from build123d import *

# Parameters (mm, degrees)
F1_DEPTH = 1.5875
F2_W     = 15.875
F2_H     = 3.175
F3_DEPTH = 2.38125
F5_W     = 12.7
F5_H     = 3.175
F6_DEPTH = 0.79375
F7_R     = 1.5875


# Not quite as in the source:
# - a feature of the source that left no trace in its solid (it failed there, or was rolled back) is left out


with BuildPart() as f1:
    # F0 (on Top) → F1 (new body)
    with BuildSketch(Plane.XY):
        Polygon((28.575, -6.35), (28.575, 6.35), (6.35, 6.35), (4.7625, 12.7), (-4.7625, 12.7), (-6.35, 6.35), (-28.575, 6.35), (-28.575, -6.35), align=None)
    extrude(amount=F1_DEPTH)

    # F2 (on face) → F3 (join)
    with BuildSketch(Plane.XY.offset(1.5875)):
        Rectangle(F2_W, F2_H)
    extrude(amount=F3_DEPTH)

    # F5 (on offset) → F6 (cut)
    with BuildSketch(Plane.XY.offset(2.38125)):
        Rectangle(F5_W, F5_H)
    extrude(amount=-F6_DEPTH, mode=Mode.SUBTRACT)

    # F7
    f7_edges = [f1.edges().sort_by_distance(p)[0] for p in [
        (-28.575, -6.35, 0.79375),
        (28.575, -6.35, 0.79375),
        (28.575, 6.35, 0.79375),
        (4.7625, 12.7, 0.79375),
        (-28.575, 6.35, 0.79375),
        (-4.7625, 12.7, 0.79375),
        (-6.35, 6.35, 0.79375),
        (6.35, 6.35, 0.79375),
    ]]
    fillet(f7_edges, radius=F7_R)


solid = f1.part
The listing builds one solid part. Answer for the finished solid, in the listing's coordinates (mm). A direction names the side the tool comes from. Give positions to 0.01 mm unless a question says otherwise; leave off trailing zeros. Write each loop counter-clockwise with the first axis right and the second up, starting at its lowest first coordinate (ties: lowest second). Pieces come first, ordered by that corner, then holes. Notation, with made-up numbers: (55.25, 35) - (64.25, 35) arc R15 ccw to (64.25, 58) - close; hole circle Ø1 at (-29, 59). An arc over 180 degrees is marked (long way). Use a Markdown table: item, result.
1. A tool of negligible diameter and unlimited length cuts with its end or side. For faces 4 (the flat face through (17, 6.35, 1)), 5 (the flat face through (-17, 6.35, 1)), 6 (the flat face through (0, -1.588, 3)), 7 (the flat face through (-7.938, 0, 3)), from which of +Z, -Z, +X, -X, +Y, -Y can it reach the whole face along a straight path? Write none if from no direction.
Values follow:
| item | result |
|---|---|
| face 4 | +Z, -Z, +X, +Y |
| face 5 | +Z, -Z, -X, +Y |
| face 6 | +Z, +X, -X, -Y |
| face 7 | +Z, -X, +Y, -Y |
2. Find the intervals of material crossed by probe 1 along Y at (x, z) = (-22, 1.25); probe 2 along X at (y, z) = (1, 3.85); probe 3 along Z at (x, y) = (-15.5, -1), in increasing order. Write a range as from..to.
Values follow:
| item | result |
|---|---|
| probe 1 | y = -6.35..6.35 |
| probe 2 | x = -7.94..7.94 |
| probe 3 | z = 0..1.59 |
3. For a pull along X with two mould halves and no side action, classify faces 1 (the flat face through (0, 1.588, 3)), 2 (the flat face through (7.938, 0, 3)), 3 (the flat face through (0, 0, 2.381)) as released by +X, released by -X, zero draft, split by the parting line, or undercut.
Values follow:
| item | result |
|---|---|
| face 1 | zero draft |
| face 2 | released by +X |
| face 3 | undercut |
4. Section D-D on y = 4.25 is taken. Write down the section's boundary in (x, z) (1 decimal), plus the area to 3 significant figures.
Values follow:
| item | result |
|---|---|
| outline | (-28.6, 0) - (28.6, 0) - (28.6, 1.6) - (-28.6, 1.6) - close |
| area | 90.7 mm² |
5. Section A-A on x = -2.5 is taken. Write down the section's boundary in (y, z).
Values follow:
| item | result |
|---|---|
| outline | (-6.35, 0) - (12.7, 0) - (12.7, 1.59) - (-6.35, 1.59) - close; (-1.59, 2.38) - (1.59, 2.38) - (1.59, 3.97) - (-1.59, 3.97) - close |
6. Each of these flat-tipped pins is pushed along its axis until it touches: P1, Ø0.5, axis at x = 19.5, z = 0.5, coming from the +Y side; P2, Ø1.5, axis at x = -8, y = 3, coming from the +Z side; P3, Ø0.7, axis at y = -0.5, z = 3, coming from the +X side; P4, Ø2.5, axis at x = 2, y = 1, coming from the -Z side. Where does it stop, or does it pass through?
Values follow:
| item | result |
|---|---|
| P1 | stops at y = 6.35 |
| P2 | stops at z = 1.59 |
| P3 | stops at x = 7.94 |
| P4 | stops at z = 0 |
